Can you work these out from the drawing? Everything is in mm from the part's minimum corner. Give positions to 0.01 mm unless a question says otherwise; leave off trailing zeros. Loops run counter-clockwise (first coordinate to the right, second up) from the corner with the lowest first, then second, coordinate; pieces in that order, holes last. Notation, with made-up numbers: (-20.5, 47.25) -> (-14.5, 47.25) arc R18 ccw to (-14.5, 70.25) -> close; hole circle Ø1 at (86.5, 7). An arc over 180 degrees is marked (long way). Return JSON: item names as keys, results as strings. Group by question number.
Q1. Suppose I cut it at B-B, the plane z = 42. Please give me the cut outline in (x, y).
Q2. Suppose I cut it at D-D, the plane x = 60.5. Please give me the cut outline in (y, z).
Q3. Suppose I cut it at A-A, the plane x = 45. Please give me the cut outline in (y, z).
Q4. Suppose I cut it at C-C, the plane y = 1.4. Count the separate pieces of the cut face and the enclosed holes in it, and give its area (3 significant figures).
Q5. Will these pins go through, and if not, where does the flat tip stop? pin 1 (3 mm diameter, centred on x = 6.55, z = 29.04, fed in from +Y); pin 2 (1 mm diameter, centred on y = 1, z = 36, fed in from -X).
Q6. I need wall thicknesses on line 1 along Z through (x, y) = (45, 0.6); line 2 along X through (y, z) = (0.5, 13); line 3 along Z through (x, y) = (30, 1.6). Which ranges of each line are inside material? Lowest first, please. Write a range as [from, to].
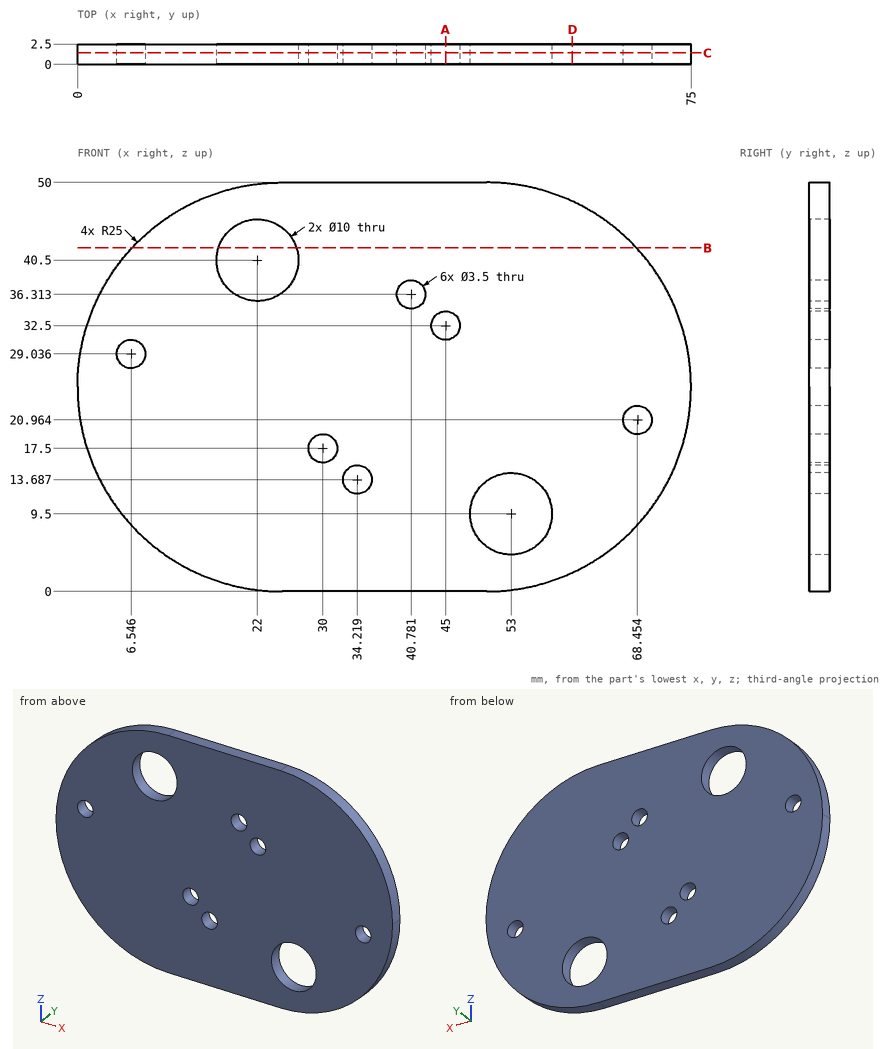
Ans:
{
 "1": {"outline": "(6.67, 0) -> (17.23, 0) -> (17.23, 2.5) -> (6.67, 2.5) -> close; (26.77, 0) -> (68.33, 0) -> (68.33, 2.5) -> (26.77, 2.5) -> close"},
 "2": {"outline": "(0, 2.31) -> (2.5, 2.31) -> (2.5, 47.69) -> (0, 47.69) -> close"},
 "3": {"outline": "(0, 0) -> (2.5, 0) -> (2.5, 30.75) -> (0, 30.75) -> close; (0, 34.25) -> (2.5, 34.25) -> (2.5, 50) -> (0, 50) -> close"},
 "4": {"separate pieces": "1", "enclosed holes": "8", "area": "3,000 mm^2"},
 "5": {"pin 1": "passes through", "pin 2": "stops at x = 2.31"},
 "6": {"line 1": "z = [0, 30.75], [34.25, 50]", "line 2": "x = [3.07, 32.61], [35.83, 49.43], [56.57, 71.93]", "line 3": "z = [0, 15.75], [19.25, 50]"}
}
